from build123d import *

# Parameters (mm, degrees)
F0_W     = 1200
F0_H     = 170
F1_DEPTH = 18
F3_DEPTH = 1200.001
F4_R     = 32.5
F5_DEPTH = 18.001


with BuildPart() as f1:
    # F0 (on Front) → F1 (new body)
    with BuildSketch(Plane.XZ):
        with Locations((600, 85)):
            Rectangle(F0_W, F0_H)
    extrude(amount=F1_DEPTH)

    # F2 (on face) → F3 (cut, through all)
    with BuildSketch(Plane.YZ.offset(1200)):
        Polygon((-18, 152), (0, 170), (-18, 170), align=None)
        Polygon((-18, 0), (0, 0), (0, 18), align=None)
    extrude(amount=-F3_DEPTH, mode=Mode.SUBTRACT)

    # F4 (on face) → F5 (cut, through all)
    with BuildSketch(Plane.XZ.offset(18)):
        with Locations((150, 76)):
            Circle(F4_R)
        with Locations((1050, 76)):
            Circle(F4_R)
        with BuildLine():
            Line((540, 51), (660, 51))
            ThreePointArc((660, 51), (663.535534, 52.464466), (665, 56))
            Line((665, 56), (665, 96))
            ThreePointArc((665, 96), (663.535534, 99.535534), (660, 101))
            Line((660, 101), (540, 101))
            ThreePointArc((540, 101), (536.464466, 99.535534), (535, 96))
            Line((535, 96), (535, 56))
            ThreePointArc((535, 56), (536.464466, 52.464466), (540, 51))
        make_face()
    extrude(amount=-F5_DEPTH, mode=Mode.SUBTRACT)


solid = f1.part
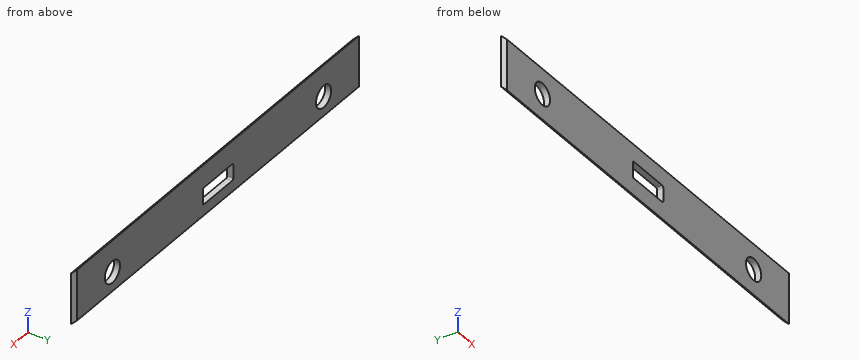
Input: part model. Units: mm. Frame: model coordinates. Round coordinates to 2 decimals unless told otherwise and drop trailing zeros. Loops run counter-clockwise (first coordinate to the right, second up) from the corner with the lowest first, then second, coordinate; pieces in that order, holes last. Notation, with made-up numbers: (-20.75, -22.75) -> (-11.75, -22.75) arc R25 ccw to (-11.75, -1.75) -> close; hole circle Ø6 at (61.25, 74.25). An arc over 180 degrees is marked (long way). Answer as a JSON object with one key per item and string values. Group by question number.
1) Pin query (flat end, axial travel): pin 1 (4 mm diameter, centred on x = 784.5, y = -7.5, fed in from +Z); pin 2 (9 mm diameter, centred on x = 581, y = -5.5, fed in from -Z); pin 3 (4 mm diameter, centred on x = 580, y = -11.5, fed in from -Z). Return the tip coordinate at first contact, or that it passes through.
2) Section query B-B on y = -9.5. Output: boundary loops of the cut face in (x, z).
3) Section query A-A on z = 76. Output: boundary loops of the cut face in (x, y), plus the area to 3 significant figures.
4) Section query D-D on x = 795. Output: boundary loops of the cut face in (y, z), plus the area to 3 significant figures.
5) Section query C-C on x = 150. Output: boundary loops of the cut face in (y, z).
6) Ray query, L1, parallel to X at y = -2.5, z = 73.5; L2, parallel to X at y = -14.75, z = 86; L3, parallel to Z at x = 149, y = -12.5. Return the intervals inside material, ascending.
Reply:
{
 "1": {"pin 1": "stops at z = 164.5", "pin 2": "stops at z = 8", "pin 3": "stops at z = 4.5"},
 "2": {"outline": "(0, 8.5) -> (1200, 8.5) -> (1200, 160.5) -> (0, 160.5) -> close; hole circle Ø65 at (150, 76); hole (535, 56) arc R5 ccw to (540, 51) -> (660, 51) arc R5 ccw to (665, 56) -> (665, 96) arc R5 ccw to (660, 101) -> (540, 101) arc R5 ccw to (535, 96) -> close; hole circle Ø65 at (1050, 76)"},
 "3": {"outline": "(0, -18) -> (117.5, -18) -> (117.5, 0) -> (0, 0) -> close; (182.5, -18) -> (535, -18) -> (535, 0) -> (182.5, 0) -> close; (665, -18) -> (1017.5, -18) -> (1017.5, 0) -> (665, 0) -> close; (1082.5, -18) -> (1200, -18) -> (1200, 0) -> (1082.5, 0) -> close", "area": "16,900 mm2"},
 "4": {"outline": "(-18, 0) -> (0, 18) -> (0, 170) -> (-18, 152) -> close", "area": "2,740 mm2"},
 "5": {"outline": "(-18, 0) -> (0, 18) -> (0, 43.5) -> (-18, 43.5) -> close; (-18, 108.5) -> (0, 108.5) -> (0, 170) -> (-18, 152) -> close"},
 "6": {"L1": "x = 0 to 117.6, 182.4 to 535, 665 to 1017.6, 1082.4 to 1200", "L2": "x = 0 to 119.08, 180.92 to 535, 665 to 1019.08, 1080.92 to 1200", "L3": "z = 5.5 to 43.52, 108.48 to 157.5"}
}
